Model file for the job. Use its own axes, mm. Face numbers are marked on the shaded views. A direction names the side the tool comes from. Give positions to 0.01 mm unless a question says otherwise; leave off trailing zeros. Loops run counter-clockwise (first coordinate to the right, second up) from the corner with the lowest first, then second, coordinate; pieces in that order, holes last. Notation, with made-up numbers: M 5.25,18 L 25.25,18 A22 ccw 25.25,50 Z; hole C 47.5,-12 d3. An arc over 180 degrees is marked long. Answer in a Markdown table with one row per item.
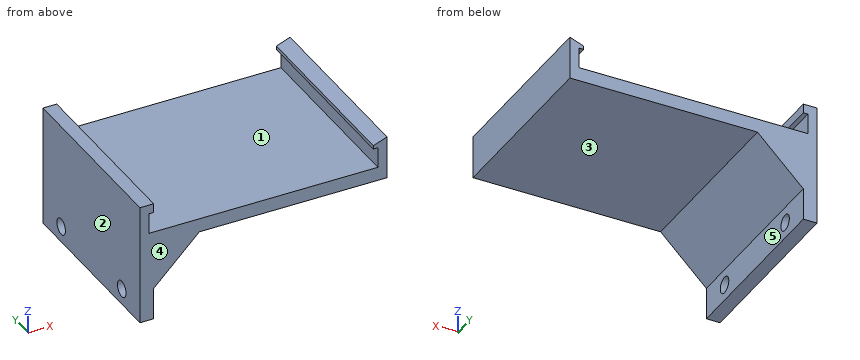
```python
from build123d import *

# Parameters (mm, degrees)
F1_DEPTH = 40
F2_SIZE  = 10
F3_R     = 1.765
F3_R_2   = 1.75
F4_DEPTH = 25


with BuildPart() as f1:
    # F0 (on Front) → F1 (new body)
    with BuildSketch(Plane.XZ):
        Polygon((0, 6.5), (0, 0), (0, -20), (3, -20), (3, -3), (54, -3), (54, 0), (54, 6.395918), (51, 5.27192), (51, 4.5), (52, 4.5), (52, 0), (2, 0), (2, 4.5), (3, 4.5), (3, 6.5), align=None)
    extrude(amount=F1_DEPTH)

    # F2
    f2_edges = [f1.edges().sort_by_distance(p)[0] for p in [
        (3, -20, -3),
    ]]
    chamfer(f2_edges, length=F2_SIZE)

    # F3 (on face) → F4 (cut)
    with BuildSketch(Plane.YZ.offset(3)):
        with Locations((-32.5, -16.5)):
            Circle(F3_R)
        with Locations((-7.5, -16.5)):
            Circle(F3_R_2)
    extrude(amount=-F4_DEPTH, mode=Mode.SUBTRACT)


solid = f1.part
```
Q1. Drop flat-ended pins along their axis: pin 1 (5.5 mm diameter, centred on y = -19, z = -15.5, fed in from +X); pin 2 (0.8 mm diameter, centred on x = 51.5, y = -20, fed in from -Z); pin 3 (12 mm diameter, centred on y = -22, z = -17, fed in from +X). Give the stop position or say it passes through.
Reported:
| item | result |
|---|---|
| pin 1 | x = 3.25 |
| pin 2 | z = -3 |
| pin 3 | x = 5 |
Q2. 3-axis set-ups, long thin cutter, end or side, ignore diameter. For the marked faces 4 and 5: which of +Z, -Z, +X, -X, +Y, -Y reach the whole face in a straight line?
Reported:
| item | result |
|---|---|
| face 4 | +Z, -Z, +X, -X, -Y |
| face 5 | -Z, +X, +Y, -Y |
Q3. Saw through at D-D (y = -32.5). Give the cut face in (x, z) (3 decimals).
Reported:
| item | result |
|---|---|
| outline | M 0,-20 L 3,-20 L 3,-18.265 L 0,-18.265 Z; M 0,-14.735 L 3,-14.735 L 3,-13 L 13,-3 L 54,-3 L 54,6.396 L 51,5.272 L 51,4.5 L 52,4.5 L 52,0 L 2,0 L 2,4.5 L 3,4.5 L 3,6.5 L 0,6.5 Z |
Q4. Saw through at B-B (z = -16.5). Give the cut face in (x, y) (3 decimals).
Reported:
| item | result |
|---|---|
| outline | M 0,-40 L 3,-40 L 3,-34.265 L 0,-34.265 Z; M 0,-30.735 L 3,-30.735 L 3,-9.25 L 0,-9.25 Z; M 0,-5.75 L 3,-5.75 L 3,0 L 0,0 Z |
Q5. Saw through at A-A (y = -7.5). Give the cut face in (x, z).
Reported:
| item | result |
|---|---|
| outline | M 0,-20 L 3,-20 L 3,-18.25 L 0,-18.25 Z; M 0,-14.75 L 3,-14.75 L 3,-13 L 13,-3 L 54,-3 L 54,6.4 L 51,5.27 L 51,4.5 L 52,4.5 L 52,0 L 2,0 L 2,4.5 L 3,4.5 L 3,6.5 L 0,6.5 Z |
Q6. Probe probe 1 along Z at (x, y) = (1.9, -32.5) (3 decimals); probe 2 along X at (y, z) = (-2.5, 2.25); probe 3 along X at (y, z) = (-15.5, 5). List the from-to ranges inside material, lowest first.
Reported:
| item | result |
|---|---|
| probe 1 | -20 to -18.265, -14.735 to 6.5 |
| probe 2 | 0 to 2, 52 to 54 |
| probe 3 | 0 to 3, 51 to 54 |
Q7. Mould opens along X. For the marked faces 1, 2 and 3 say: released by +X, released by -X, zero draft, split by the parting line, or undercut.
Reported:
| item | result |
|---|---|
| face 1 | undercut |
| face 2 | released by -X |
| face 3 | zero draft |
Q8. Saw through at C-C (y = -3). Give the cut face in (x, z).
Reported:
| item | result |
|---|---|
| outline | M 0,-20 L 3,-20 L 3,-13 L 13,-3 L 54,-3 L 54,6.4 L 51,5.27 L 51,4.5 L 52,4.5 L 52,0 L 2,0 L 2,4.5 L 3,4.5 L 3,6.5 L 0,6.5 Z |
